```python
from build123d import *

# Parameters (mm, degrees)
EXTRUDE_1_DEPTH          = 30
CUT_EXTRUDE_1_DEPTH      = 73.256487598
CUT_EXTRUDE_1_DEPTH_BACK = 73.256487598
SKETCH_2_R               = 2
SKETCH_3_R               = 2.75
CUT_EXTRUDE_2_DEPTH      = 73.256487598


with BuildPart() as part:
    # 草图1 → 凸台-拉伸1 (new, symmetric)
    with BuildSketch(Plane.XY):
        Polygon((0, 0), (15, 0), (15, -64), (0, -64), (0, -61), (12, -61), (12, -3), (0, -3), align=None)
    extrude(amount=EXTRUDE_1_DEPTH, both=True)

    # 草图2 → 切除-拉伸1 (cut, two sides: drawn at the far end of the back side and taken through both)
    with BuildSketch(Plane(origin=(0, 0, 0), x_dir=(1, 0, 0), z_dir=(0, 1, 0)).offset(-CUT_EXTRUDE_1_DEPTH_BACK)):
        with Locations(Location((6, 22.5, 0), (0, 0, 270))):
            Circle(SKETCH_2_R)
        with Locations(Location((6, -22.5, 0), (0, 0, 270))):
            Circle(SKETCH_2_R)
    extrude(amount=CUT_EXTRUDE_1_DEPTH + CUT_EXTRUDE_1_DEPTH_BACK, mode=Mode.SUBTRACT)

    # 草图3 → 切除-拉伸2 (cut, through all)
    with BuildSketch(Plane(origin=(15, 0, 0), x_dir=(0, 0, -1), z_dir=(1, 0, 0))):
        with Locations(Location((-22.5, -32, 0), (0, 0, 90))):
            Circle(SKETCH_3_R)
        with Locations(Location((22.5, -32, 0), (0, 0, 90))):
            Circle(SKETCH_3_R)
    extrude(amount=-CUT_EXTRUDE_2_DEPTH, mode=Mode.SUBTRACT)


solid = part.part
```
Could you check a few things on this model? Use its own coordinates, in mm. A direction names the side the tool comes from. Coordinates: 2 decimals unless noted, no trailing zeros. Loops run counter-clockwise (first coordinate to the right, second up) from the corner with the lowest first, then second, coordinate; pieces in that order, holes last. Notation, with made-up numbers: M -15,12.25 L 3,12.25 A9 ccw 3,29.25 Z; hole C 65,14.25 d6. An arc over 180 degrees is marked long. Put each result on its own line as item: value. Start each with the question number.
(1) Suppose I cut it at D-D on y = -32. Please give me the cut outline in (x, z).
(2) For faces 1 (the face through (12, -32, 0)), 2 (the face through (13.521, -34.747, 22.621)), which set-ups out of +Z, -Z, +X, -X, +Y, -Y let a thin tool reach every point of the face, with its end or its side?
(3) Suppose I cut it at C-C on x = 6. Please give me the cut outline in (y, z).
(4) Thinking about a two-plate mould opening in Y: for faces 3 (the face through (7, 0, 0)), 4 (the face through (7.352, -62.521, -23.974)), 5 (the face through (8, -64, 0)), 6 (the face through (6, -61, 0)), which applies, pulls with the +Y half, pulls with the -Y half, needs draft (parallel to the pull), parting line crosses it, or undercut?
(5) I need wall thicknesses on line 1 (Z direction, x = 13.7, y = -32); line 2 (Z direction, x = 6, y = -0.9); line 3 (Y direction, x = 5.75, z = 0). Which ranges of each line are inside material? Lowest first, please. Write a range as from..to.
(6) Suppose I cut it at A-A on x = 10. Please give me the cut outline in (y, z).
(7) Suppose I cut it at B-B on z = 22.5. Please give me the cut outline in (x, y), then the cut area to 4 significant figures.
Solutions:
1. outline: M 12,-30 L 15,-30 L 15,-25.25 L 12,-25.25 Z; M 12,-19.75 L 15,-19.75 L 15,19.75 L 12,19.75 Z; M 12,25.25 L 15,25.25 L 15,30 L 12,30 Z
2. face 1: +Z, -Z, -X
2. face 2: +X, -X
3. outline: M -64,-30 L -61,-30 L -61,-24.5 L -64,-24.5 Z; M -64,-20.5 L -61,-20.5 L -61,20.5 L -64,20.5 Z; M -64,24.5 L -61,24.5 L -61,30 L -64,30 Z; M -3,-30 L 0,-30 L 0,-24.5 L -3,-24.5 Z; M -3,-20.5 L 0,-20.5 L 0,20.5 L -3,20.5 Z; M -3,24.5 L 0,24.5 L 0,30 L -3,30 Z
4. face 3: pulls with the +Y half
4. face 4: needs draft
4. face 5: pulls with the -Y half
4. face 6: undercut
5. line 1: z = -30..-25.25, -19.75..19.75, 25.25..30
5. line 2: z = -30..-24.5, -20.5..20.5, 24.5..30
5. line 3: y = -64..-61, -3..0
6. outline: M -64,-30 L -61,-30 L -61,30 L -64,30 Z; M -3,-30 L 0,-30 L 0,30 L -3,30 Z
7. outline: M 0,-64 L 4,-64 L 4,-61 L 0,-61 Z; M 0,-3 L 4,-3 L 4,0 L 0,0 Z; M 8,-64 L 15,-64 L 15,-34.75 L 12,-34.75 L 12,-61 L 8,-61 Z; M 8,-3 L 12,-3 L 12,-29.25 L 15,-29.25 L 15,0 L 8,0 Z
7. area: 223.5 mm2
